```python
from build123d import *

# Parameters (mm, degrees)
BOSS_EXTRUDE1_DEPTH           = 50.8
CUT_EXTRUDE1_DEPTH            = 38.1
CUT_EXTRUDE2_DEPTH            = 38.1
BOSS_EXTRUDE3_DEPTH           = 12.7
BOSS_EXTRUDE3_DEPTH_BACK      = 12.7
SKETCH16_R                    = 9.525
F_5_16_18_TAPPED_HOLE4_REACH  = 170.58
F_5_16_18_TAPPED_HOLE4_BORE_R = 3.2639
BOSS_EXTRUDE6_DEPTH           = 12.7
BOSS_EXTRUDE6_DEPTH_BACK      = 5.08
SKETCH20_R                    = 9.525
F_5_16_18_TAPPED_HOLE5_REACH  = 180.939
F_5_16_18_TAPPED_HOLE5_BORE_R = 3.2639


with BuildPart() as part:
    # Sketch1 → Boss-Extrude1 (new body)
    with BuildSketch(Plane(origin=(0, 0, 0), x_dir=(1, 0, 0), z_dir=(0, 1, 0))):
        with BuildLine():
            ThreePointArc((25.4, 43.994090512), (-50.8, 0), (25.4, -43.994090512))
            ThreePointArc((25.4, -43.994090512), (101.6, 0), (25.4, 43.994090512))
        make_face()
    extrude(amount=BOSS_EXTRUDE1_DEPTH)

    # Sketch3 → Cut-Extrude1 (cut)
    with BuildSketch(Plane(origin=(0, 50.8, 0), x_dir=(1, 0, 0), z_dir=(0, 1, 0))):
        with BuildLine():
            ThreePointArc((25.4, -28.398063314), (88.9, 0), (25.4, 28.398063314))
            ThreePointArc((25.4, 28.398063314), (-38.1, 0), (25.4, -28.398063314))
        make_face()
    extrude(amount=-CUT_EXTRUDE1_DEPTH, mode=Mode.SUBTRACT)

    # Sketch5 → Cut-Extrude2 (cut)
    with BuildSketch(Plane(origin=(0, 12.7, 0), x_dir=(1, 0, 0), z_dir=(0, 1, 0))):
        Polygon((63.5, 0), (57.15, 10.998522628), (44.45, 10.998522628), (38.1, 0), (44.45, -10.998522628), (57.15, -10.998522628), align=None)
        Polygon((12.7, 0), (6.35, 10.998522628), (-6.35, 10.998522628), (-12.7, 0), (-6.35, -10.998522628), (6.35, -10.998522628), align=None)
    extrude(amount=-CUT_EXTRUDE2_DEPTH, mode=Mode.SUBTRACT)

    # Sketch16 → Boss-Extrude3 (add, two sides: drawn at the far end of the back side and taken through both)
    with BuildSketch(Plane(origin=(-17.374623281, 0, -47.736385136), x_dir=(0, -1, 0), z_dir=(-0.34202014332566666, 0, -0.9396926207859091)).offset(-BOSS_EXTRUDE3_DEPTH_BACK)):
        with Locations(Location((-31.75, 0, 0), (0, 0, 270))):
            Circle(SKETCH16_R)
    extrude(amount=BOSS_EXTRUDE3_DEPTH + BOSS_EXTRUDE3_DEPTH_BACK)

    # 5/16-18 Tapped Hole4 bore (on position points) → 5/16-18 Tapped Hole4 (cut, up to next)
    with BuildSketch(Plane(origin=(-21.718279101, 31.75, -59.67048142), x_dir=(-0.939692620786, 0, 0.342020143326), z_dir=(-0.342020143326, 0, -0.939692620786)), mode=Mode.PRIVATE) as f_5_16_18_tapped_hole4_sk1:
        Circle(F_5_16_18_TAPPED_HOLE4_BORE_R)
    f_5_16_18_tapped_hole4_tool1 = extrude(f_5_16_18_tapped_hole4_sk1.sketch, amount=-F_5_16_18_TAPPED_HOLE4_REACH, mode=Mode.PRIVATE) & part.part
    add(f_5_16_18_tapped_hole4_tool1.solids().sort_by_distance((-21.718279, 31.75, -59.670481))[0], mode=Mode.SUBTRACT)

    # Sketch20 → Boss-Extrude6 (add, two sides: drawn at the far end of the back side and taken through both)
    with BuildSketch(Plane(origin=(30.54220241, 0, 65.497964437), x_dir=(0, -1, 0), z_dir=(0.42261826174068773, 0, 0.9063077870366555)).offset(-BOSS_EXTRUDE6_DEPTH_BACK)):
        with Locations(Location((-31.75, 46.040435581, 0), (0, 0, 90))):
            Circle(SKETCH20_R)
    extrude(amount=BOSS_EXTRUDE6_DEPTH + BOSS_EXTRUDE6_DEPTH_BACK)

    # 5/16-18 Tapped Hole5 bore (on position points) → 5/16-18 Tapped Hole5 (cut, up to next)
    with BuildSketch(Plane(origin=(77.636259621, 31.75, 57.550544477), x_dir=(0.906307787037, 0, -0.422618261741), z_dir=(0.422618261741, 0, 0.906307787037)), mode=Mode.PRIVATE) as f_5_16_18_tapped_hole5_sk1:
        Circle(F_5_16_18_TAPPED_HOLE5_BORE_R)
    f_5_16_18_tapped_hole5_tool1 = extrude(f_5_16_18_tapped_hole5_sk1.sketch, amount=-F_5_16_18_TAPPED_HOLE5_REACH, mode=Mode.PRIVATE) & part.part
    add(f_5_16_18_tapped_hole5_tool1.solids().sort_by_distance((77.63626, 31.75, 57.550544))[0], mode=Mode.SUBTRACT)


solid = part.part
```
For this review, take the finished solid that the model builds, in its own axes (mm). A direction names the side the tool comes from. Round coordinates to 2 decimals unless told otherwise and drop trailing zeros. Loops run counter-clockwise (first coordinate to the right, second up) from the corner with the lowest first, then second, coordinate; pieces in that order, holes last.
(1) We need section B-B (y = 37). Give the boundary of the cut face in (x, z), plus the area to 3 significant figures.
Returned:
outline: (-29.19, -56.95) - (-14.25, -62.39) - (-9.69, -49.87) arc R50.8 ccw to (25.4, -43.99) arc R50.8 ccw to (79.21, 42.11) - (84.84, 54.19) - (70.43, 60.91) - (64.8, 48.83) arc R50.8 ccw to (25.4, 43.99) arc R50.8 ccw (long way) to (-24.63, -44.43) - close; hole (25.4, -28.4) arc R38.1 ccw (long way) to (25.4, 28.4) arc R38.1 ccw (long way) to start
area: 5,330 mm2
(2) Tool access review of faces 4 (the flat face through (9.57, 6.44, -5.42)), 5 (the cylindrical face through (-38.08, 32.02, -1.23)), 6 (the cylindrical face through (-20.5, 22.3, -52.8)): name each direction out of +Z, -Z, +X, -X, +Y, -Y from which nothing blocks a thin tool from reaching the whole face with its end or side.
Returned:
face 4: +Y, -Y
face 5: +Y
face 6: none
(3) We need section D-D (x = 2.5). Give the boundary of the cut face in (y, z).
Returned:
outline: (0, -50.74) - (50.8, -50.74) - (50.8, -38.02) - (12.7, -38.02) - (12.7, -11) - (0, -11) - close; (0, 11) - (12.7, 11) - (12.7, 38.02) - (50.8, 38.02) - (50.8, 50.74) - (0, 50.74) - close
(4) Wall thickness on line 1 along Z through (x, y) = (50, 28); line 2 along X through (y, z) = (14.5, 32); line 3 along Y through (x, z) = (29, 12): over which ranges is each line inside the solid? List them lowest first.
Returned:
line 1: z = -50.79 to -38.09, 38.09 to 50.79
line 2: x = -39.45 to -20.68, 20.68 to 30.12, 71.48 to 90.25
line 3: y = 0 to 12.7
(5) We need section C-C (z = 23.5). Give the boundary of the cut face in (x, y).
Returned:
outline: (-45.04, 0) - (95.84, 0) - (95.84, 50.8) - (80.79, 50.8) - (80.79, 12.7) - (-29.99, 12.7) - (-29.99, 50.8) - (-45.04, 50.8) - close
(6) Mouldability with a two-part tool opening along X and no side actions: class faces 1 (the flat face through (-9.48, 6.44, -5.58)), 2 (the flat face through (81.35, 31.88, 55.82)), 3 (the flat face through (24, 0, -1)) as released by +X, released by -X, zero draft, split by the parting line, or undercut.
Returned:
face 1: undercut
face 2: released by +X
face 3: zero draft
(7) Clearance check with flat-ended pins moving along their axes: P1, Ø4, axis at x = 50.5, y = 5.5, coming from the -Z side; P2, Ø10, axis at x = 52, y = 11.5, coming from the +Z side; P3, Ø6, axis at y = 18.5, z = -42.5, coming from the -X side. State where each tip first meets the part, or that it passes through.
Returned:
P1: stops at z = -50.8
P2: stops at z = 50.8
P3: stops at x = -31.94
(8) We need section A-A (x = 50.8). Give the boundary of the cut face in (y, z), plus the area to 3 significant figures.
Returned:
outline: (0, -50.8) - (50.8, -50.8) - (50.8, -38.1) - (12.7, -38.1) - (12.7, -11) - (0, -11) - close; (0, 11) - (12.7, 11) - (12.7, 38.1) - (50.8, 38.1) - (50.8, 50.8) - (0, 50.8) - close
area: 1,980 mm2
